The listing builds one solid part. Answer for the finished solid, in the listing's coordinates (mm). A direction names the side the tool comes from. Round coordinates to 2 decimals unless told otherwise and drop trailing zeros. Order: outer loops, then holes, each group sorted by start corner. A loop starts at its lowest first (then second) coordinate and runs counter-clockwise, first axis right, second up. Notation, with made-up numbers: (38.25, 12) -> (69.25, 12) arc R31 ccw to (69.25, 40) -> close; hole circle Ø9 at (22, 46.25). An arc over 180 degrees is marked (long way). Return JSON: item names as keys, results as strings. Group by question number.
(1) The part is cut by section C-C (x = 1.5). Determine the outline of the cut face in (y, z) (3 decimals), plus the area to 3 significant figures.
(2) The part is cut by section A-A (y = 0). Determine the outline of the cut face in (x, z) (3 decimals), plus the area to 3 significant figures.
(3) Determine the mould class of faces 1 (the face through (5, -9, 2)), 2 (the face through (2.5, 1.2, 2.5)), 3 (the face through (1.233, 2.175, 2.487)), 4 (the face through (2, 0, 0)) for opening direction Z: +Z half, -Z half, draft (parallel to the pull), parting line (faces both ways), or undercut.
(4) The part is cut by section D-D (z = 1.85). Determine the outline of the cut face in (x, y), plus the area to 3 significant figures.
(5) Consider line 1 (Y direction, x = 2.65, z = 2.5) (3 decimals); line 2 (Z direction, x = 2.85, y = 0) (3 decimals); line 3 (Y direction, x = 4, z = 2.3). Determine where each line is inside the solid, lowest interval first. Write a range as [from, to].
(6) Which of the six approach directions +Z, -Z, +X, -X, +Y, -Y give full straight-line access (tool end or side, diameter ignored) to faces 5 (the face through (2.291, 8.516, 2.367)), 6 (the face through (1, -2, 3.4)), 7 (the face through (5, -3, 2))?
(7) The part is cut by section B-B (x = 3.75). Determine the outline of the cut face in (y, z) (3 decimals), plus the area to 3 significant figures.
(8) Each of these flat-tipped pins is pushed along its axis until it touches: pin 1 (1.5 mm diameter, centred on y = -5, z = 1.5, fed in from +X); pin 2 (1.6 mm diameter, centred on y = 7.5, z = 2.5, fed in from -X); pin 3 (1 mm diameter, centred on y = -1, z = 2.5, fed in from -X); pin 4 (0.5 mm diameter, centred on y = 1, z = 2.5, fed in from -X). Where does it stop, or does it pass through?
Autodesk Inventor part; units mm, degrees
ref_plane "YZ Plane" through (0, 0, 0) normal (1, 0, 0) x (0, 1, 0)
ref_plane "XZ Plane" through (0, 0, 0) normal (0, 1, 0) x (-1, 0, 0)
ref_plane "XY Plane" through (0, 0, 0) normal (0, 0, 1) x (1, 0, 0)
sketch "Sketch1" plane through (0, 0, 0) normal (0, 0, 1) x (1, 0, 0)
  line L0 (10, -10) -> (-10, -10)
  line L1 (-10, -10) -> (-10, 10)
  line L2 (-10, 10) -> (10, 10)
  line L3 (10, 10) -> (10, -10)
  line L4 (10, -10) -> (-10, 10) construction
  line L5 (-10, -10) -> (10, 10) construction
  line L6 (10, -10) -> (6, -10)
  line L7 (6, -10) -> (6, 10)
  line L8 (6, 10) -> (10, 10)
  line L9 (10, 10) -> (10, -10)
  line L10 (6, 2) -> (4, 2)
  line L11 (4, 2) -> (4, -2)
  line L12 (4, -2) -> (6, -2)
  line L13 (6, -2) -> (6, 2)
  line L14 (0, 10) -> (0, -10)
  point P0 (0, 0)
  dimension "d0" = 20
  dimension "d1" = 20
  dimension "d2" = 4
  dimension "d6" = 2
  dimension "d7" = 2
  dimension "d8" = 4
  dimension "d9" = 2
  dimension "d44" = 6
extrude "Extrusion1" add sketch "Sketch1" along normal blind 5 contours L0 L14 L2 L7 L10 L11 L12
ref_plane "Work Plane1" through (0, 0, 2.5) normal (0, 0, 1) x (1, 0, 0)
sketch "Sketch2" plane through (0, 0, 2.5) normal (0, 0, 1) x (1, 0, 0)
  line L0 (0, 10) -> (0, -10)
  line L1 (0, 2.8868) -> (2.5, 1.4434)
  line L2 (2.5, 1.4434) -> (2.5, -1.4434)
  line L3 (2.5, -1.4434) -> (0, -2.8868)
  line L4 (0, -2.8868) -> (-2.5, -1.4434)
  line L5 (-2.5, -1.4434) -> (-2.5, 1.4434)
  line L6 (-2.5, 1.4434) -> (0, 2.8868)
  point P0 (0, 0)
  point P1 (0, 0)
  dimension "d12" = 5
extrude "Extrusion2" cut sketch "Sketch2" along normal mid plane 1.8
sketch "Sketch3" plane through (0, 0, 5) normal (0, 0, 1) x (1, 0, 0)
  circle A0 centre (0, 0) radius 1.75
  dimension "d15" = 3.5
extrude "Extrusion3" cut sketch "Sketch3" against normal blind 8
sketch "Sketch4" plane through (0, 10, 0) normal (-1, 0, 0) x (0, 0, 1)
  circle A0 centre (2.5, -2.5) radius 1.025
  circle A1 centre (2.5, -17.5) radius 1.025
  line L0 (0, 0) -> (5, 0)
  line L1 (0, 0) -> (0, -8.25)
  line L2 (0, -11.75) -> (0, -20)
  line L3 (0, -20) -> (5, -20)
  point P0 (0, -10)
  dimension "d18" = 2.05
  dimension "d19" = 2.05
  dimension "d20" = 2.5
  dimension "d21" = 2.5
  dimension "d22" = 2.5
  dimension "d23" = 2.5
extrude "Extrusion4" cut sketch "Sketch4" against normal blind 25
sketch "Sketch5" plane through (0, 0, 0) normal (0, 0, -1) x (-1, 0, 0)
  line L0 (-4, -2) -> (-4, 2)
  line L1 (-6, -10) -> (-6, -2)
  line L2 (-4, 2) -> (-6, 2)
  line L3 (-6, 2) -> (-6, -2)
  line L4 (-6, -2) -> (-4, -2)
  line L5 (-4, -2) -> (-4, 2)
  point P0 (0, 0)
extrude "Extrusion5" add sketch "Sketch5" against normal blind 5
sketch "Sketch6" plane through (0, 0, 0) normal (0, 0, -1) x (-1, 0, 0)
  line L0 (-6, -10) -> (-6, 10)
  circle A0 centre (-6, 6) radius 2.5
  line L1 (-6, -9) -> (-3.5, -9)
  line L2 (-3.5, -9) -> (-3.5, -3)
  line L3 (-3.5, -3) -> (-6, -3)
  line L4 (-6, -3) -> (-6, -9)
  line L5 (0, -10) -> (-6, -10)
  line L6 (-6, 10) -> (0, 10)
  point P0 (0, 0)
  point P1 (-6, 8.5)
  point P2 (-6, 3.5)
  dimension "d32" = 2.5
  dimension "d33" = 1
  dimension "d34" = 6
  dimension "d35" = 5
  dimension "d36" = 4
extrude "Extrusion6" cut sketch "Sketch6" against normal blind 5 contours L0 A0 | L0 L3 L2 L1 picked at (-5.3485, 6.5196)
sketch "Sketch7" plane through (6, -3, 0) normal (1, 0, 0) x (0, 0, -1)
  circle A0 centre (-2.5, 3) radius 1.025
  line L0 (-5, 0) -> (-5, 6.5)
  line L1 (0, -7) -> (-5, -7)
  point P0 (0, 3)
  dimension "d39" = 2.5
  dimension "d40" = 10
  dimension "d41" = 2.05
extrude "Extrusion7" cut sketch "Sketch7" against normal blind 12
equation "\"d18\" = d19"
properties part number "POMSliderMotor"
Answer below:
{
 "1": {"outline": "(-10, 0) -> (-0.901, 0) -> (-0.901, 1.6) -> (-2.021, 1.6) -> (-2.021, 3.4) -> (-0.901, 3.4) -> (-0.901, 5) -> (-10, 5) -> close; (0.901, 0) -> (10, 0) -> (10, 5) -> (0.901, 5) -> (0.901, 3.4) -> (2.021, 3.4) -> (2.021, 1.6) -> (0.901, 1.6) -> close; hole circle Ø2.05 at (-7.5, 2.5); hole circle Ø2.05 at (7.5, 2.5)", "area": "80.4 mm²"},
 "2": {"outline": "(1.75, 0) -> (6, 0) -> (6, 1.475) -> (1.75, 1.475) -> close; (1.75, 3.525) -> (6, 3.525) -> (6, 5) -> (1.75, 5) -> close", "area": "12.5 mm²"},
 "3": {"face 1": "draft", "face 2": "undercut", "face 3": "undercut", "face 4": "-Z half"},
 "4": {"outline": "(0, -10) -> (6, -10) -> (6, -9) -> (3.5, -9) -> (3.5, -8.29) -> (0, -8.29) -> close; (0, -6.71) -> (3.5, -6.71) -> (3.5, -3) -> (6, -3) -> (6, -0.79) -> (2.5, -0.79) -> (2.5, -1.44) -> (0, -2.89) -> close; (0, 2.89) -> (2.5, 1.44) -> (2.5, 0.79) -> (6, 0.79) -> (6, 3.5) arc R2.5 cw to (3.6, 6.71) -> (0, 6.71) -> close; (0, 8.29) -> (5, 8.29) arc R2.5 cw to (6, 8.5) -> (6, 10) -> (0, 10) -> close", "area": "66.8 mm²"},
 "5": {"line 1": "y = [-10, -8.525], [-6.475, -1.025], [1.025, 6.475], [8.525, 10]", "line 2": "z = [0, 1.475], [3.525, 5]", "line 3": "y = [-10, -9], [-3, -1.01], [1.01, 4.5], [8.51, 10]"},
 "6": {"face 5": "+X, -X", "face 6": "-X", "face 7": "+Z, -Z, +X"},
 "7": {"outline": "(-10, 0) -> (-9, 0) -> (-9, 5) -> (-10, 5) -> close; (-3, 0) -> (4.91, 0) -> (4.91, 5) -> (-3, 5) -> close; (7.09, 0) -> (10, 0) -> (10, 5) -> (7.09, 5) -> (7.09, 3.439) arc R1.025 cw (long way) to (7.09, 1.561) -> close; hole circle Ø2.05 at (0, 2.5)", "area": "53.3 mm²"},
 "8": {"pin 1": "stops at x = 3.5", "pin 2": "passes through", "pin 3": "stops at x = 2.4", "pin 4": "stops at x = 2.5"}
}
